from build123d import *

# Parameters (mm, degrees)
F0_R          = 4
F0_R_2        = 3
F1_DEPTH      = 50
F2_R          = 6
F3_DEPTH      = 25
F3_DEPTH_BACK = 25
F5_DEPTH      = 15
F6_SIZE       = 0.1
F7_R          = 0.9999
F8_R          = 3
F9_DEPTH      = 2
F9_DEPTH_BACK = 60
F12_R         = 2
F13_DEPTH     = 15
F14_SIZE      = 1
F15_R         = 10
F16_DEPTH     = 5
F17_R         = 10
F17_R_2       = 3.75
F18_DEPTH     = 1
F20_SIZE      = 1


# Not quite as in the source:
# - a fillet or chamfer that OpenCascade refuses, or shapes differently, is made with other operations: its cross-section is extruded or revolved along the edge and cut away or added
# - a fillet or chamfer is up to 0.001 mm smaller than in the source, because OpenCascade refuses the exact size


with BuildPart() as f1:
    # F0 (on Front) → F1 (new body)
    with BuildSketch(Plane.XZ):
        Circle(F0_R)
        Circle(F0_R_2, mode=Mode.SUBTRACT)
    extrude(amount=F1_DEPTH)

    # F2 (on Right) → F3 (cut, two sides)
    with BuildSketch(Plane.YZ) as f3_sk:
        with Locations((-5, 8.5)):
            Circle(F2_R)
    extrude(amount=-F3_DEPTH, mode=Mode.SUBTRACT)
    extrude(f3_sk.sketch, amount=F3_DEPTH_BACK, mode=Mode.SUBTRACT)

    # F4 (on face) → F5 (cut)
    with BuildSketch(Plane(origin=(0, 0, 0), x_dir=(-1, 0, 0), z_dir=(0, 1, 0))):
        Polygon((-4.3, 1), (-4.3, 0), (-4.3, -1), (-3.3, -1), (-3.3, 1), align=None)
        Polygon((1, -3.3), (-1, -3.3), (-1, -4.3), (0, -4.3), (1, -4.3), align=None)
        Polygon((3.3, 1), (3.3, -1), (4.3, -1), (4.3, 0), (4.3, 1), align=None)
    extrude(amount=-F5_DEPTH, mode=Mode.SUBTRACT)

    # F6
    f6_edges = [f1.edges().sort_by_distance(p)[0] for p in [
        (0, 0, 4),
        (2.828427, 0, -2.828427),
        (-2.828427, 0, -2.828427),
    ]]
    chamfer(f6_edges, length=F6_SIZE)

    # F7 (radius 1 in the source; OpenCascade refuses exactly that, so slightly less here)
    f7_edges = [f1.edges().sort_by_distance(p)[0] for p in [
        (3.586492, -15, 1),
        (3.586492, -15, -1),
        (1, -15, -3.586492),
        (-1, -15, -3.586492),
        (-3.586492, -15, -1),
        (-3.586492, -15, 1),
    ]]
    fillet(f7_edges, radius=F7_R)

    # F8 (on face) → F9 (join, two sides)
    with BuildSketch(Plane(origin=(0, 0, 0), x_dir=(-1, 0, 0), z_dir=(0, 1, 0))) as f9_sk:
        Circle(F8_R)
    extrude(amount=F9_DEPTH)
    extrude(f9_sk.sketch, amount=-F9_DEPTH_BACK)

    # F10: chamfer of 2 x 0.1398536239 on 1 edges, made by hand


with BuildPart() as f10_tool2:
    # F10_s3 → F10_t4 (revolve)
    with BuildSketch(Plane.XY):
        Polygon((-3, 0), (-2.8601463761, 2), (-3, 2), align=None)
    revolve(axis=Axis((0, 2, 0), (0, 1, 0)))

    split(bisect_by=Plane.XZ, keep=Keep.BOTTOM)


with BuildPart() as f1_1:
    add(f1.part)

    # F10_t1: cut F10_tool2
    add(f10_tool2.part, mode=Mode.SUBTRACT)

    # F12 (on face) → F13 (join)
    with BuildSketch(Plane(origin=(0, 2, 0), x_dir=(-1, 0, 0), z_dir=(0, 1, 0))):
        Circle(F12_R)
    extrude(amount=F13_DEPTH)

    # F14
    f14_edges = [f1_1.edges().sort_by_distance(p)[0] for p in [
        (2, 17, 0),
    ]]
    chamfer(f14_edges, length=F14_SIZE)

    # F15 (on face) → F16 (join)
    with BuildSketch(Plane(origin=(0, 2, 0), x_dir=(-1, 0, 0), z_dir=(0, 1, 0))):
        Circle(F15_R)
    extrude(amount=F16_DEPTH)

    # F17 (on face) → F18 (join)
    with BuildSketch(Plane.XZ.offset(-2)):
        Circle(F17_R)
        Circle(F17_R_2, mode=Mode.SUBTRACT)
    extrude(amount=F18_DEPTH)

    # F20
    f20_edges = [f1_1.edges().sort_by_distance(p)[0] for p in [
        (10, 7, 0),
    ]]
    chamfer(f20_edges, length=F20_SIZE)


solid = f1_1.part
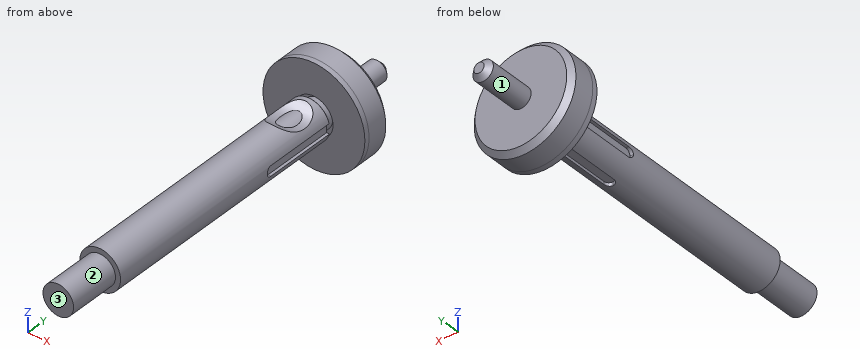
Read the model definition and answer for the solid it produces. Units are mm, in the model's axes. Face numbers are marked on the shaded views. A direction names the side the tool comes from. Give positions to 0.01 mm unless a question says otherwise; leave off trailing zeros. Write each loop counter-clockwise with the first axis right and the second up, starting at its lowest first coordinate (ties: lowest second). Pieces come first, ordered by that corner, then holes. Notation, with made-up numbers: M -21.75,-12 L 24.25,-12 A30 cw 24.25,22 Z; hole C 42.5,15.25 d4. An arc over 180 degrees is marked long. One line per item, written item: value. Start each with the question number.
(1) Flat-ended cylindrical pins translate along their axes: pin 1 Ø0.5 at (y, z) = (-7.5, -3.5) entering from -X; pin 2 Ø1 at (y, z) = (-7.5, 0) entering from -X; pin 3 Ø0.5 at (x, y) = (-3.5, -8.5) entering from -Z. Find the tip coordinate at first contact, or state that the pin passes through.
(2) A tool of negligible diameter and unlimited length cuts with its end or side. For the marked faces 1, 2 and 3, from which of +Z, -Z, +X, -X, +Y, -Y can it reach the whole face along a straight path? Write none if from no direction.
(3) Find section B-B (y = 11.5). Determine the outline of the cut face in (x, z), plus the area to 3 significant figures.
(4) Find section A-A (y = -44). Determine the outline of the cut face in (x, z).
(5) Find the intervals of material crossed by line 1 (Z direction, x = 0, y = 1.6); line 2 (Y direction, x = 6, z = 5.5); line 3 (Y direction, x = -3.5, z = 0.75), in increasing order.
Results below:
1. pin 1: stops at x = -2.33
1. pin 2: stops at x = -3.3
1. pin 3: stops at z = -2.33
2. face 1: +Y
2. face 2: -Y
2. face 3: +Z, -Z, +X, -X, -Y
3. outline: C 0,0 d4
3. area: 12.6 mm^2
4. outline: C 0,0 d8
5. line 1: z = -10 to -3.75, -2.89 to 2.89, 3.75 to 10
5. line 2: y = 1 to 7
5. line 3: y = -50 to -14.66, 2 to 7
